Geometry: final body of the model. Coordinates: model frame, mm. A direction names the side the tool comes from. Round coordinates to 2 decimals unless told otherwise and drop trailing zeros. Order: outer loops, then holes, each group sorted by start corner. A loop starts at its lowest first (then second) coordinate and runs counter-clockwise, first axis right, second up. Notation, with made-up numbers: M 85,6.5 L 124,6.5 A22 cw 124,45.5 Z; hole C 49.5,68 d7. An arc over 180 degrees is marked long. Return JSON: item names as keys, results as strings. Group by question number.
Q1. Contact query for flat-ended pins moving along their axis: pin 1 (10 mm diameter, centred on x = -13, z = 29.5, fed in from +Y); pin 2 (2.5 mm diameter, centred on y = 1.5, z = 20, fed in from +X); pin 3 (2.5 mm diameter, centred on y = 2.5, z = 2, fed in from -X); pin 4 (2 mm diameter, centred on y = 1, z = -25.5, fed in from -X). Output: stop coordinate, or through.
Q2. Cut plane C-C on x = -7. Output: boundary loops of the cut face in (y, z), and give its area (3 significant figures).
Q3. Cut plane D-D on z = 9. Output: boundary loops of the cut face in (x, y).
Q4. Access query for faces 4 (the face through (-3.75, 2, -19)), 5 (the face through (-19, 2, 7.5)), 6 (the face through (30, 2, -22.5)), 7 (the face through (-26.25, 2, -23)). Directions: +Z, -Z, +X, -X, +Y, -Y. A direction counts if a zero-diameter tool reaches every point of the face in a straight line with its end or side. Return the directions, or none.
Q5. Mould query, pull axis Z, two halves, no side actions, for faces 1 (the face through (-5, 5, 0)), 2 (the face through (-30, 2, 22.5)), 3 (the face through (11.25, 2, 8)). Classes: released by +Z, released by -Z, zero draft, split by the parting line, or undercut.
Q6. Ray query, probe 1 along Z at (x, y) = (-16, 3.9); probe 2 along X at (y, z) = (0.8, -19.5); probe 3 along Z at (x, y) = (16.5, 4.8). Return the intervals inside material, ascending.
Q7. Cut plane A-A on z = 28. Output: boundary loops of the cut face in (x, y).
Q8. Cut plane B-B on x = 5. Output: boundary loops of the cut face in (y, z), and give its area (3 significant figures).
```python
from build123d import *

# Parameters (mm, degrees)
SKETCH1_W           = 22.5
SKETCH1_H           = 30
SKETCH1_W_2         = 7.5
SKETCH1_H_2         = 7.5
BOSS_EXTRUDE1_DEPTH = 5
CUT_EXTRUDE1_DEPTH  = 51.698249477


with BuildPart() as part:
    # Sketch1 → Boss-Extrude1 (new body)
    with BuildSketch(Plane(origin=(0, 0, 0), x_dir=(1, 0, 0), z_dir=(0, 1, 0))):
        Polygon((-11.25, 7.5), (-11.25, 15), (-18.75, 15), (-18.75, 37.5), (-26.25, 37.5), (-26.25, 7.5), align=None)
        Rectangle(SKETCH1_W, SKETCH1_H)
        with Locations((0, 18.75)):
            Rectangle(SKETCH1_W_2, SKETCH1_H_2)
        Polygon((26.25, 15), (11.25, 15), (11.25, 7.5), (33.75, 7.5), (33.75, 22.5), (26.25, 22.5), align=None)
        Polygon((11.25, -22.5), (11.25, -15), (3.75, -15), (3.75, -30), (18.75, -30), (18.75, -37.5), (26.25, -37.5), (26.25, -22.5), align=None)
        Polygon((-18.75, -15), (-11.25, -15), (-11.25, -7.5), (-26.25, -7.5), (-26.25, -22.5), (-33.75, -22.5), (-33.75, -30), (-18.75, -30), align=None)
    extrude(amount=BOSS_EXTRUDE1_DEPTH)

    # Sketch2 → Cut-Extrude1 (cut, through all)
    with BuildSketch(Plane(origin=(0, 5, 0), x_dir=(1, 0, 0), z_dir=(0, 1, 0))):
        Polygon((0, 5.625), (-1.396218154, 1.327882373), (-5.914475011, 1.327882373), (-2.259128429, -1.327882373), (-3.655346583, -5.625), (0, -2.969235253), (3.655346583, -5.625), (2.259128429, -1.327882373), (5.914475011, 1.327882373), (1.396218154, 1.327882373), align=None)
    extrude(amount=-CUT_EXTRUDE1_DEPTH, mode=Mode.SUBTRACT)


solid = part.part
```
Result sheet:
{
 "1": {"pin 1": "passes through", "pin 2": "stops at x = 11.25", "pin 3": "stops at x = -11.25", "pin 4": "stops at x = -26.25"},
 "2": {"outline": "M 0,-15 L 5,-15 L 5,15 L 0,15 Z", "area": "150 mm²"},
 "3": {"outline": "M -26.25,0 L 11.25,0 L 11.25,5 L -26.25,5 Z"},
 "4": {"face 4": "-Z, +Y, -Y", "face 5": "-X, +Y, -Y", "face 6": "-Z, +X, +Y, -Y", "face 7": "-Z, -X, +Y, -Y"},
 "5": {"face 1": "zero draft", "face 2": "released by -Z", "face 3": "undercut"},
 "6": {"probe 1": "z = -15 to -7.5, 7.5 to 15", "probe 2": "x = -26.25 to -18.75, -3.75 to 3.75, 26.25 to 33.75", "probe 3": "z = -15 to -7.5, 22.5 to 30"},
 "7": {"outline": "M -33.75,0 L -18.75,0 L -18.75,5 L -33.75,5 Z; M 3.75,0 L 26.25,0 L 26.25,5 L 3.75,5 Z"},
 "8": {"outline": "M 0,-15 L 5,-15 L 5,-1.33 L 0,-1.33 Z; M 0,-0.66 L 5,-0.66 L 5,30 L 0,30 Z", "area": "222 mm²"}
}
